from build123d import *

# Parameters (mm, degrees)
F1_DEPTH = 460
F2_W     = 30
F2_H     = 93
F3_DEPTH = 20
F5_DEPTH = 20
F6_R     = 3.25
F7_DEPTH = 15.001


with BuildPart() as f1:
    # F0 (on Front) → F1 (new body)
    with BuildSketch(Plane.XZ):
        Polygon((18.685265, 56.099155), (-11.314735, 38.215565), (-11.314735, -50.784435), (18.685265, -50.784435), (18.685265, -35.784435), (18.685265, 38.636174), (18.685265, 44.457167), (16.12505, 42.930973), (3.685265, 35.515373), (3.685265, 38.636174), (3.685265, 41.336367), (18.685265, 50.278161), align=None)
    extrude(amount=F1_DEPTH)

    # F2 (on face) → F3 (cut)
    with BuildSketch(Plane.XZ.offset(460)):
        with Locations((3.685265, 10.715565)):
            Rectangle(F2_W, F2_H)
    extrude(amount=-F3_DEPTH, mode=Mode.SUBTRACT)

    # F4 (on face) → F5 (cut)
    with BuildSketch(Plane(origin=(0, 0, 0), x_dir=(-1, 0, 0), z_dir=(0, 1, 0))):
        Polygon((-18.685265, 57.215565), (-18.685265, -35.784435), (11.314735, -35.784435), (11.314735, -26.784435), (11.314735, 57.215565), align=None)
    extrude(amount=-F5_DEPTH, mode=Mode.SUBTRACT)

    # F6 (on face) → F7 (cut, through all)
    with BuildSketch(Plane.XY.offset(-35.784435)):
        with Locations((3.685265, -10)):
            Circle(F6_R)
        with Locations((3.685265, -450)):
            Circle(F6_R)
    extrude(amount=-F7_DEPTH, mode=Mode.SUBTRACT)


solid = f1.part
Design review of the part built by this model. Coordinates are the model's own, in mm. A direction names the side the tool comes from. Round coordinates to 2 decimals unless told otherwise and drop trailing zeros. Loops run counter-clockwise (first coordinate to the right, second up) from the corner with the lowest first, then second, coordinate; pieces in that order, holes last. Notation, with made-up numbers: M 16.5,25.5 L 50.5,25.5 A31 ccw 50.5,55.5 Z; hole C -34.5,-37 d10. An arc over 180 degrees is marked long. Answer as a JSON object with one key per item and string values.
Item 1: Wall thickness on L1, parallel to Y at x = 4, z = -42; L2, parallel to X at y = -450, z = -43; L3, parallel to Y at x = -4, z = 42: over which ranges is each line inside the solid? List them lowest first. Write a range as from..to.
Answer sheet:
{"L1": "y = -460..-453.23, -446.77..-13.23, -6.77..0", "L2": "x = -11.31..0.44, 6.94..18.69", "L3": "y = -440..-20"}
Item 2: We need section B-B on y = -316. Give the boundary of the cut face in (x, z), and give its area (3 significant figures).
Answer sheet:
{"outline": "M -11.31,-50.78 L 18.69,-50.78 L 18.69,44.46 L 16.13,42.93 L 3.69,35.52 L 3.69,41.34 L 18.69,50.28 L 18.69,56.1 L -11.31,38.22 Z", "area": "2,850 mm^2"}
Item 3: We need section A-A on x = 12. Give the boundary of the cut face in (y, z), and give its area (3 significant figures).
Answer sheet:
{"outline": "M -460,-50.78 L 0,-50.78 L 0,-35.78 L -20,-35.78 L -20,40.47 L -440,40.47 L -440,-35.78 L -460,-35.78 Z; M -440,46.29 L -20,46.29 L -20,52.11 L -440,52.11 Z", "area": "41,400 mm^2"}
Item 4: Machinability: for faces 4 (the flat face through (3, -440, 1)), 5 (the flat face through (7.2, -9.9, -35.784)), 6 (the flat face through (3, -460, -43)), which of the approach directions +Z, -Z, +X, -X, +Y, -Y give a long, thin tool a straight path to every point of the face, cutting with its end or side? Answer none if there is none.
Answer sheet:
{"face 4": "+Z, +X, -X, -Y", "face 5": "+Z, +X, -X, +Y", "face 6": "+Z, -Z, +X, -X, -Y"}
Item 5: The part is to be moulded in two halves that separate along Z. For faces 1 (the flat face through (11.08, -227.06, 45.745)), 2 (the flat face through (3, 0, -43)), 3 (the flat face through (3.895, -227.06, 47.283)), say which applies: pulls with the +Z half, pulls with the -Z half, needs draft (parallel to the pull), parting line crosses it, or undercut.
Answer sheet:
{"face 1": "undercut", "face 2": "needs draft", "face 3": "pulls with the +Z half"}
Item 6: We need section C-C on z = 26.5. Give the boundary of the cut face in (x, y).
Answer sheet:
{"outline": "M -11.31,-440 L 18.69,-440 L 18.69,-20 L -11.31,-20 Z"}
Item 7: Clearance check with flat-ended pins moving along their axes: P1, Ø15, axis at x = 7.5, z = 21, coming from the +Y side; P2, Ø5, axis at x = 3, y = -397, coming from the +Z side; P3, Ø3, axis at x = 5.5, y = -102.5, coming from the +Z side. State where each tip first meets the part, or that it passes through.
Answer sheet:
{"P1": "stops at y = -20", "P2": "stops at z = 48.24", "P3": "stops at z = 49.13"}
